Check sheet for the drawn part. Datum: minimum x, y, z corner. Units: mm. A direction names the side the tool comes from. Round coordinates to 2 decimals unless told otherwise and drop trailing zeros. Write each loop counter-clockwise with the first axis right and the second up, starting at its lowest first coordinate (ties: lowest second). Pieces come first, ordered by that corner, then holes. Notation, with made-up numbers: M 62,-16 L 104,-16 A22 ccw 104,1 Z; hole C 48,25.25 d10. An arc over 180 degrees is marked long. Put each result on its own line as item: value.
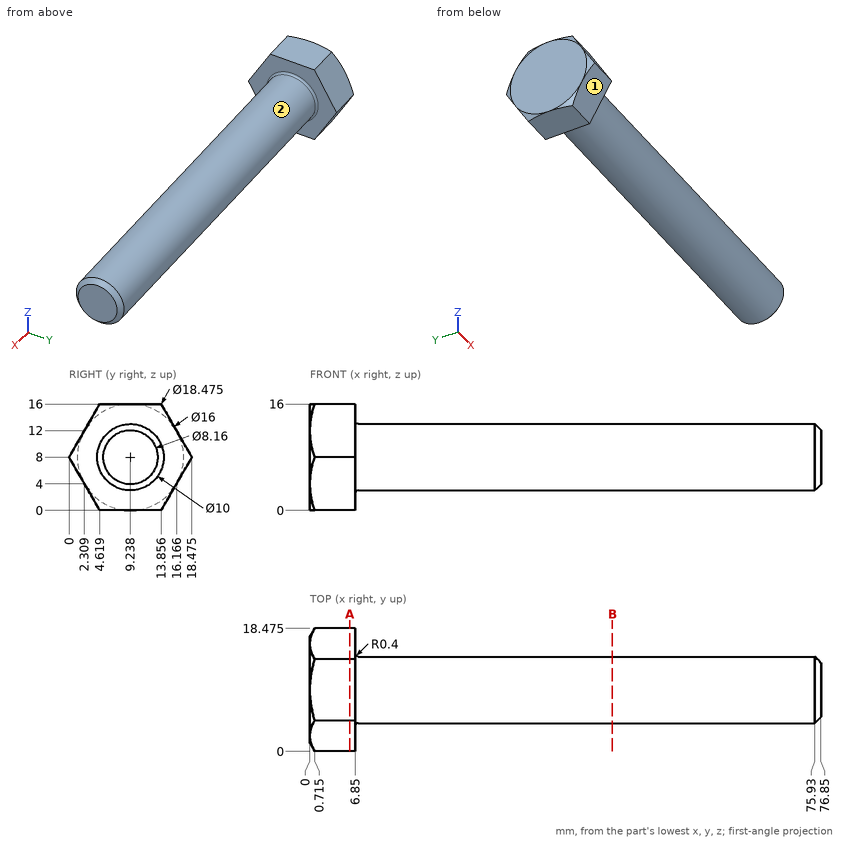
1. Cross-section at A-A (x = 6). Enter the section's corners in (y, z) (1 decimal), then the cut area to 3 significant figures.
Computed values:
outline: M 0,8 L 4.6,0 L 13.9,0 L 18.5,8 L 13.9,16 L 4.6,16 Z
area: 222 mm2
2. Access from +Z, -Z, +X, -X, +Y, -Y to the whole of each face (thin tool, end or side, straight path). Record for the marked faces 1 and 2.
Computed values:
face 1: -Z, +X, -X, -Y
face 2: +X
3. Cross-section at B-B (x = 45.5). Enter the section's corners in (y, z).
Computed values:
outline: C 9.24,8 d10
4. Depth check by flat-ended pin: pin 1 Ø6 at (x, y) = (52, 5.5) entering from -Z (1 decimal); pin 2 Ø4 at (x, y) = (16.5, 13.5) entering from +Z; pin 3 Ø6 at (x, z) = (11.5, 12) entering from +Y. Enter the tip coordinate at first touch or a pass-through.
Computed values:
pin 1: stops at z = 3.1
pin 2: stops at z = 12.46
pin 3: stops at y = 14.14
5. Scan lines: probe 1 along X at (y, z) = (11.5, 13); probe 2 along Y at (x, z) = (13.5, 8.25); probe 3 along Y at (x, z) = (46, 7). Record each from-to range of solid material in increasing order.
Computed values:
probe 1: x = 0 to 6.85
probe 2: y = 4.24 to 14.23
probe 3: y = 4.34 to 14.14
